Autodesk Inventor part; units mm, degrees
ref_plane "YZ Plane" through (0, 0, 0) normal (1, 0, 0) x (0, 1, 0)
ref_plane "XZ Plane" through (0, 0, 0) normal (0, 1, 0) x (-1, 0, 0)
ref_plane "XY Plane" through (0, 0, 0) normal (0, 0, 1) x (1, 0, 0)
sketch "スケッチ1" plane through (0, 0, 0) normal (1, 0, 0) x (0, 1, 0)
  line L0 (0, 0) -> (1, 0) construction
  line L1 (1.9, 0) -> (1.9, 1.75)
  line L2 (1.65, 2) -> (0.866, 2)
  line L3 (0, 2) -> (0, 1.5) construction
  line L4 (1, 0) -> (1, -10)
  line L5 (1, -10) -> (0, -10)
  line L6 (0, -10) -> (0, 0)
  line L7 (1, 0) -> (1.9, 0)
  line L8 (0.866, 2) -> (0.433, 1.25) construction
  line L9 (0.433, 1.25) -> (-0.433, 1.25) construction
  line L10 (-0.433, 1.25) -> (-0.866, 2) construction
  line L11 (-0.866, 2) -> (-0.433, 2.75) construction
  line L12 (-0.433, 2.75) -> (0.433, 2.75) construction
  line L13 (0.433, 2.75) -> (0.866, 2) construction
  line L14 (0.866, 2) -> (0, 1.5)
  line L15 (0.866, 2) -> (0, 2) construction
  line L16 (0, 1.5) -> (0, 0)
  arc A0 (1.9, 1.75) -> (1.65, 2) centre (1.65, 1.75) ccw
  dimension "d0" = 1.5
  dimension "d1" = 3.8
  dimension "d2" = 2
  dimension "d3" = 10
  dimension "d4" = 2
  dimension "d6" = 0.25
  dimension "d11" = 30
revolve "回転1" add sketch "スケッチ1" angle 360 about axis through (0, 0, 1.5) along (0, 0, -1)
sketch "スケッチ2" plane through (0, 0, 2) normal (0, 0, 1) x (1, 0, 0)
  line L0 (0.866, 0) -> (0.433, -0.75)
  line L1 (0.433, -0.75) -> (-0.433, -0.75)
  line L2 (-0.433, -0.75) -> (-0.866, 0)
  line L3 (-0.866, 0) -> (-0.433, 0.75)
  line L4 (-0.433, 0.75) -> (0.433, 0.75)
  line L5 (0.433, 0.75) -> (0.866, 0)
  point P0 (0, 0)
  point P1 (0, 0)
  dimension "d8" = 1.5
extrude "押し出し1" cut sketch "スケッチ2" against normal blind 1
chamfer "面取り1" distance 0.25 angle 45 1 edges at (0, -1, -10)
properties part number "10_053_CAP_BOLT_M2X10_R1" material "鋼、炭素鋼"
Here's how the part is built. I have some questions about the finished solid (model axes, mm). A direction names the side the tool comes from. Coordinates: 2 decimals unless noted, no trailing zeros. Order: outer loops, then holes, each group sorted by start corner. A loop starts at its lowest first (then second) coordinate and runs counter-clockwise, first axis right, second up.
1) Which directions (+Z, -Z, +X, -X, +Y, -Y) give clear straight access to the entire face, cutting with the end or side of a thin tool? Please do faces 1 (the face through (-1, 1, 2)), 2 (the face through (-1, 0, -5)), 3 (the face through (0, 0.75, 1.5)).
2) Will these pins go through, and if not, where does the flat tip stop? pin 1 (2 mm diameter, centred on x = 1.5, z = -4.5, fed in from +Y); pin 2 (1.5 mm diameter, centred on x = 1, z = -8, fed in from -Y); pin 3 (1.6 mm diameter, centred on x = 0, y = 0, fed in from +Z).
3) We'd pull the mould along X, two halves only. Please class faces 4 (the face through (-0.08, -1.9, 0.89)), 5 (the face through (-1, 1, 0)), 6 (the face through (0, 0, 1)): +X half, -X half, draft (parallel to the pull), parting line (faces both ways), or undercut.
4) Imagine slicing it at B-B on z = 0.25. List the corners of the cut face in (x, y) for me, and give its area (3 significant figures).
5) I need wall thicknesses on line 1 (Z direction, x = 1.25, y = 0.7); line 2 (Y direction, x = 0.9, z = -0.25); line 3 (Y direction, x = 0.5, z = -0.75). Which ranges of each line are inside material? Lowest first, please.
6) Imagine slicing it at A-A on x = 0. List the corners of the cut face in (y, z) for me.
7) Imagine slicing it at C-C on z = -3.5. List the corners of the cut face in (x, y) for me.
Response values:
1. face 1: +Z, +X, -X, +Y, -Y
1. face 2: -Z
1. face 3: +Z
2. pin 1: stops at y = 0.87
2. pin 2: stops at y = -0.97
2. pin 3: stops at z = 1.96
3. face 4: parting line
3. face 5: draft
3. face 6: undercut
4. outline: circle Ø3.8 at (0, 0)
4. area: 11.3 mm2
5. line 1: z = 0 to 2
5. line 2: y = -0.44 to 0.44
5. line 3: y = -0.87 to 0.87
6. outline: (-1.9, 0) - (-1, 0) - (-1, -9.75) - (-0.75, -10) - (0.75, -10) - (1, -9.75) - (1, 0) - (1.9, 0) - (1.9, 1.75) arc R0.25 ccw to (1.65, 2) - (0.87, 2) - (0.75, 1.93) - (0.75, 1) - (-0.75, 1) - (-0.75, 1.93) - (-0.87, 2) - (-1.65, 2) arc R0.25 ccw to (-1.9, 1.75) - close
7. outline: circle Ø2 at (0, 0)
